Read the model definition and answer for the solid it produces. Units are mm, in the model's axes. A direction names the side the tool comes from. Give positions to 0.01 mm unless a question says otherwise; leave off trailing zeros. Write each loop counter-clockwise with the first axis right and the second up, starting at its lowest first coordinate (ties: lowest second). Pieces come first, ordered by that corner, then holes. Notation, with made-up numbers: M 49.5,-25.75 L 98.5,-25.75 A34 cw 98.5,7.25 Z; hole C 56,-15.5 d3. An arc over 180 degrees is marked long. Use a Markdown table: item, result. Add a question column.
Item 1: A cutting plane is placed at B-B on x = 12.7. Count the separate pieces of the cut face and the enclosed holes in it, then the cut area to 3 significant figures.
Item 2: Consider probe 1 along Y at (x, z) = (6.25, 100.5) (1 decimal); probe 2 along X at (y, z) = (5.75, 221.5); probe 3 along Z at (x, y) = (12.7, 7) (3 decimals). Determine where each line is inside the solid, lowest interval first. Write a range as [from, to].
Item 3: Given P1, Ø2, axis at x = 22, y = 5, coming from the +Z side; P2, Ø1.3, axis at x = 11, y = 8.5, coming from the +Z side; P3, Ø1.3, axis at x = 2.5, y = 4.5, coming from the -Z side, each flat-ended and moving along its own axis, determine where each tip first touches the part or whether it passes through.
Item 4: For faces 1 (the flat face through (1.38, 5.89, 13.71)), 2 (the flat face through (1.587, 5, 122)), 3 (the flat face through (18.225, 0.783, 15.831)), determine the directions among +Z, -Z, +X, -X, +Y, -Y from which every point of the face is accessible in a straight line to the end or side of a thin tool.
Item 5: The mould has two halves that part along X. Classify faces 4 (the flat face through (13, 7.938, 118)), 5 (the flat face through (13, 0, 121)), 6 (the flat face through (25.4, 5, 121)): pulls with the +X half, pulls with the -X half, needs draft (parallel to the pull), parting line crosses it, or undercut.
Item 6: A cutting plane is placed at A-A on z = 210. Determine the outline of the cut face in (x, y) (1 decimal).
from build123d import *

# Parameters (mm, degrees)
SKETCH1_W           = 25.4
SKETCH1_H           = 9.525
BOSS_EXTRUDE1_DEPTH = 228.6
SKETCH2_W           = 22.225
SKETCH2_H           = 6.35
CUT_EXTRUDE1_DEPTH  = 231.203921828
CUT_EXTRUDE2_DEPTH  = 231.203921828
CUT_EXTRUDE3_DEPTH  = 231.203921828
BOSS_EXTRUDE2_DEPTH = 9.525
SKETCH6_R           = 9.525
CUT_EXTRUDE4_DEPTH  = 9.525


with BuildPart() as part:
    # Sketch1 → Boss-Extrude1 (new body)
    with BuildSketch(Plane.XY):
        with Locations((12.7, 4.7625)):
            Rectangle(SKETCH1_W, SKETCH1_H)
    extrude(amount=BOSS_EXTRUDE1_DEPTH)

    # Sketch2 → Cut-Extrude1 (cut, through all)
    with BuildSketch(Plane.XY.offset(228.6)):
        with Locations((12.7, 4.7625)):
            Rectangle(SKETCH2_W, SKETCH2_H)
    extrude(amount=-CUT_EXTRUDE1_DEPTH, mode=Mode.SUBTRACT)

    # Sketch3 → Cut-Extrude2 (cut, through all)
    with BuildSketch(Plane.XZ):
        Polygon((20.032348419, 12.7), (16.366174209, 19.05), (9.033825791, 19.05), (5.367651581, 12.7), (9.033825791, 6.35), (16.366174209, 6.35), align=None)
    extrude(amount=-CUT_EXTRUDE2_DEPTH, mode=Mode.SUBTRACT)

    # Sketch4 → Cut-Extrude3 (cut, through all)
    with BuildSketch(Plane(origin=(0, 9.525, 0), x_dir=(1, 0, 0), z_dir=(0, 1, 0))):
        Polygon((25.4, -15.875), (17.4625, -3.432478139), (7.9375, -3.432478139), (0, -15.875), (0, 0), (25.4, 0), align=None)
    extrude(amount=-CUT_EXTRUDE3_DEPTH, mode=Mode.SUBTRACT)

    # Sketch5 → Boss-Extrude2 (add)
    with BuildSketch(Plane(origin=(0, 9.525, 0), x_dir=(1, 0, 0), z_dir=(0, 1, 0))):
        with BuildLine():
            Line((0, -228.6), (25.4, -228.6))
            ThreePointArc((25.4, -228.6), (12.7, -241.3), (0, -228.6))
        make_face()
    extrude(amount=-BOSS_EXTRUDE2_DEPTH)

    # Sketch6 → Cut-Extrude4 (cut)
    with BuildSketch(Plane(origin=(0, 9.525, 0), x_dir=(1, 0, 0), z_dir=(0, 1, 0))):
        with Locations(Location((12.7, -228.6, 0), (0, 0, 270))):
            Circle(SKETCH6_R)
    extrude(amount=-CUT_EXTRUDE4_DEPTH, mode=Mode.SUBTRACT)


solid = part.part
Filled in:
| question | item | result |
|---|---|---|
| 1 | separate pieces | 5 |
| 1 | enclosed holes | 0 |
| 1 | area | 675 mm² |
| 2 | probe 1 | [0, 1.6], [7.9, 9.5] |
| 2 | probe 2 | [0, 1.59], [23.81, 25.4] |
| 2 | probe 3 | [238.125, 241.3] |
| 3 | P1 | z = 238.21 |
| 3 | P2 | z = 241.26 |
| 3 | P3 | z = 228.6 |
| 4 | face 1 | -Z, -X, +Y, -Y |
| 4 | face 2 | -Z |
| 4 | face 3 | +Y, -Y |
| 5 | face 4 | undercut |
| 5 | face 5 | needs draft |
| 5 | face 6 | pulls with the +X half |
| 6 | outline | M 0,0 L 25.4,0 L 25.4,9.5 L 0,9.5 Z; hole M 1.6,1.6 L 23.8,1.6 L 23.8,7.9 L 1.6,7.9 Z |
